Verification items for the finished model (mm, model axes). Face numbers are marked on the shaded views. A direction names the side the tool comes from. Coordinates: 2 decimals unless noted, no trailing zeros. Order: outer loops, then holes, each group sorted by start corner. A loop starts at its lowest first (then second) coordinate and runs counter-clockwise, first axis right, second up.
Q1. Depth check by flat-ended pin: P1, Ø4, axis at y = 3, z = -1.5, coming from the +X side; P2, Ø5, axis at y = 4.5, z = -14, coming from the +X side; P3, Ø12, axis at x = -5.5, z = -10, coming from the -Y side; P4, Ø4, axis at y = -4, z = -21, coming from the -X side. Enter the tip coordinate at first touch or a pass-through.
Q2. Cross-section at C-C, the plane y = 0. Record the boundary of the cut face in (x, z).
Q3. Thickness scan on line 1 (Z direction, x = 8, y = 3); line 2 (X direction, y = -3.5, z = -4.5); line 3 (X direction, y = 0, z = 9). Record the ranges inside material, lowest first.
Q4. Cross-section at B-B, the plane x = 0. Record the boundary of the cut face in (y, z).
Q5. Cross-section at D-D, the plane z = -20. Record the boundary of the cut face in (x, y), and give its area (3 significant figures).
Q6. Set-up check for the marked faces 1 and 2: record each of +Z, -Z, +X, -X, +Y, -Y from which the full face is reachable in a straight line by a thin tool's end or side.
Q7. Cross-section at A-A, the plane z = 8.5. Record the boundary of the cut face in (x, y).
from build123d import *

# Parameters (mm, degrees)
SKETCH3_R           = 4
BOSS_EXTRUDE1_DEPTH = 12.822075


with BuildPart() as part:
    # Sketch1 → Revolve1 (revolve)
    with BuildSketch(Plane.XY):
        with BuildLine():
            Line((-23.848480035, 7.5), (-21.742814905, 7.5))
            ThreePointArc((-21.742814905, 7.5), (-23, 0), (-21.742814905, -7.5))
            Line((-21.742814905, -7.5), (-23.848480035, -7.5))
            ThreePointArc((-23.848480035, -7.5), (-25, 0), (-23.848480035, 7.5))
        make_face()
    revolve(axis=Axis((0, 8.20070368, 0), (0, -1, 0)))

    # Sketch3 → Boss-Extrude1 (add)
    with BuildSketch(Plane.XY.offset(37.5)):
        Circle(SKETCH3_R)
    boss_extrude1 = extrude(amount=-BOSS_EXTRUDE1_DEPTH)

    # Mirror1: Boss-Extrude1 across plane
    add(boss_extrude1.mirror(Plane.XY))

    # Sketch4 → Cut-Revolve1 (revolve, cut)
    with BuildSketch(Plane(origin=(0, 0, 0), x_dir=(0, 0, -1), z_dir=(1, 0, 0))):
        with BuildLine():
            Line((0, 40), (0, 37.5))
            ThreePointArc((0, 37.5), (-37.5, 0), (0, -37.5))
            Line((0, -37.5), (0, -40))
            ThreePointArc((0, -40), (-40, 0), (0, 40))
        make_face()
    revolve(axis=Axis((0, 37.5, 0), (0, -1, 0)), mode=Mode.SUBTRACT)


solid = part.part
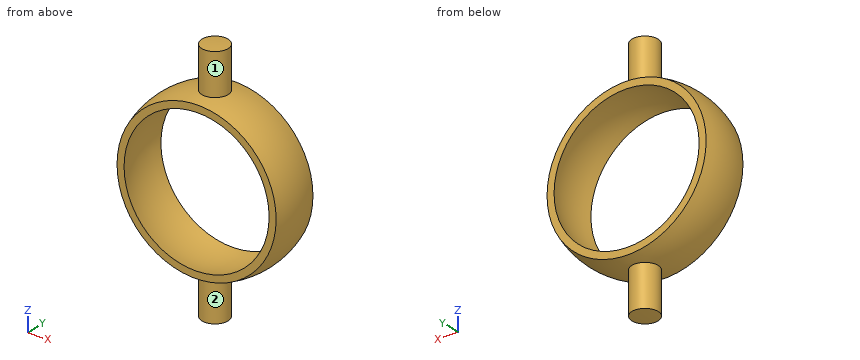
Check values:
1. P1: stops at x = 24.96
1. P2: stops at x = 21.82
1. P3: passes through
1. P4: stops at x = -15.8
2. outline: (-4, -37.29) arc R37.5 ccw to (4, -37.29) - (4, -24.68) arc R25 ccw to (4, 24.68) - (4, 37.29) arc R37.5 ccw to (-4, 37.29) - (-4, 24.68) arc R25 ccw to (-4, -24.68) - close; hole circle Ø46 at (0, 0)
3. line 1: z = -23.49 to -21.35, 21.35 to 23.49
3. line 2: x = -24.34 to -22.28, 22.28 to 24.34
3. line 3: x = -23.32 to -21.17, 21.17 to 23.32
4. outline: (-7.5, -23.85) arc R25 ccw to (-4, -24.68) - (-4, -37.29) arc R37.5 ccw to (4, -37.29) - (4, -24.68) arc R25 ccw to (7.5, -23.85) - (7.5, -21.74) arc R23 cw to (-7.5, -21.74) - close; (-7.5, 21.74) arc R23 cw to (7.5, 21.74) - (7.5, 23.85) arc R25 ccw to (4, 24.68) - (4, 37.29) arc R37.5 ccw to (-4, 37.29) - (-4, 24.68) arc R25 ccw to (-7.5, 23.85) - close
5. outline: (-12.99, -7.5) - (-8.53, -7.5) arc R11.36 cw to (-8.53, 7.5) - (-12.99, 7.5) arc R15 ccw to start; (8.53, -7.5) - (12.99, -7.5) arc R15 ccw to (12.99, 7.5) - (8.53, 7.5) arc R11.36 cw to start
5. area: 116 mm2
6. face 1: +Z
6. face 2: -Z
7. outline: (-22.28, -7.5) - (-20.01, -7.5) arc R21.37 cw to (-20.01, 7.5) - (-22.28, 7.5) arc R23.51 ccw to start; (20.01, -7.5) - (22.28, -7.5) arc R23.51 ccw to (22.28, 7.5) - (20.01, 7.5) arc R21.37 cw to start
